Geometry check sheet. Reference: the model listing, model coordinates, mm. A direction names the side the tool comes from. Round coordinates to 2 decimals unless told otherwise and drop trailing zeros. Loops run counter-clockwise (first coordinate to the right, second up) from the corner with the lowest first, then second, coordinate; pieces in that order, holes last. Notation, with made-up numbers: (33.25, -0.75) - (48.25, -0.75) arc R19 cw to (48.25, 4.25) - close; hole circle Ø2 at (47, 12.5). An arc over 180 degrees is marked (long way). Answer in a Markdown table with one row per item. Add a question column.
```python
from build123d import *

# Parameters (mm, degrees)
F0_W     = 11
F0_H     = 21
F0_W_2   = 5
F0_H_2   = 15
F1_DEPTH = 3
F2_W     = 11
F2_H     = 21
F3_DEPTH = 2
F4_R     = 2
F5_R     = 5


with BuildPart() as f1:
    # F0 (on Top) → F1 (new body)
    with BuildSketch(Plane.XY):
        Rectangle(F0_W, F0_H)
        Rectangle(F0_W_2, F0_H_2, mode=Mode.SUBTRACT)
    extrude(amount=F1_DEPTH)

    # F2 (on face) → F3 (join)
    with BuildSketch(Plane(origin=(0, 0, 0), x_dir=(1, 0, 0), z_dir=(0, 0, -1))):
        Rectangle(F2_W, F2_H)
    extrude(amount=F3_DEPTH)

    # F4
    f4_edges = [f1.edges().sort_by_distance(p)[0] for p in [
        (-2.5, -7.5, 1.5),
        (-2.5, 7.5, 1.5),
    ]]
    fillet(f4_edges, radius=F4_R)

    # F5
    f5_edges = [f1.edges().sort_by_distance(p)[0] for p in [
        (-5.5, -10.5, 0.5),
        (-5.5, 10.5, 0.5),
    ]]
    fillet(f5_edges, radius=F5_R)


solid = f1.part
```
Q1. Set-up check for faces 1 (the flat face through (1, 7.5, 1)), 2 (the flat face through (2, 10.5, 1)): record each of +Z, -Z, +X, -X, +Y, -Y from which the full face is reachable in a straight line by a thin tool's end or side.
Q2. Scan lines: line 1 (X direction, y = 3.5, z = 1.8); line 2 (Z direction, x = -2, y = -2); line 3 (Y direction, x = -1, z = 2.1). Record each from-to range of solid material in increasing order. Write a range as from..to.
Q3. Release check for a two-part mould opening along X. For faces 3 (the flat face through (5.5, 0, 1)), 4 (the flat face through (1, -7.5, 1)), 5 (the flat face through (0, 0, -2)) record: +X half, -X half, draft (parallel to the pull), parting line (faces both ways), or undercut.
Q4. Depth check by flat-ended pin: P1, Ø1.5, axis at x = -2, y = 0, coming from the +Z side; P2, Ø2.5, axis at x = -1, y = 0, coming from the +Z side; P3, Ø2, axis at x = -2.5, z = 1, coming from the -Y side. Enter the tip coordinate at first touch or a pass-through.
Q5. Cross-section at A-A, the plane z = 2. Enter the section's corners in (x, y).
Q6. Cross-section at B-B, the plane y = 0.5. Enter the section's corners in (x, z).
Q7. Cross-section at C-C, the plane x = -2. Enter the section's corners in (y, z), plus the area to 3 significant figures.
Q8. Cross-section at D-D, the plane z = -1.45. Enter the section's corners in (x, y), plus the area to 3 significant figures.
Check sheet entries:
| question | item | result |
|---|---|---|
| 1 | face 1 | +Z |
| 1 | face 2 | +Z, -Z, +X, -X, +Y |
| 2 | line 1 | -5.5..-2.5, 2.5..5.5 |
| 2 | line 2 | -2..0 |
| 2 | line 3 | -10.47..-7.44, 7.44..10.47 |
| 3 | face 3 | +X half |
| 3 | face 4 | undercut |
| 3 | face 5 | draft |
| 4 | P1 | z = 3 |
| 4 | P2 | z = 0 |
| 4 | P3 | y = -10.4 |
| 5 | outline | (-5.5, -5.5) arc R5 ccw to (-0.5, -10.5) - (5.5, -10.5) - (5.5, 10.5) - (-0.5, 10.5) arc R5 ccw to (-5.5, 5.5) - close; hole (-2.5, -5.5) arc R2 ccw to (-0.5, -7.5) - (2.5, -7.5) - (2.5, 7.5) - (-0.5, 7.5) arc R2 ccw to (-2.5, 5.5) - close |
| 6 | outline | (-5.5, -2) - (5.5, -2) - (5.5, 3) - (2.5, 3) - (2.5, 0) - (-2.5, 0) - (-2.5, 3) - (-5.5, 3) - close |
| 7 | outline | (-10.27, -2) - (10.27, -2) - (10.27, 3) - (6.82, 3) - (6.82, 0) - (-6.82, 0) - (-6.82, 3) - (-10.27, 3) - close |
| 7 | area | 61.8 mm² |
| 8 | outline | (-5.5, -5.5) arc R5 ccw to (-0.5, -10.5) - (5.5, -10.5) - (5.5, 10.5) - (-0.5, 10.5) arc R5 ccw to (-5.5, 5.5) - close |
| 8 | area | 220 mm² |
